The figure shows three views and two pictorial views of one solid part (mm, origin at its lowest corner). Answer the questions. A direction names the side the tool comes from. Coordinates: 2 decimals unless noted, no trailing zeros. Return JSON: item names as keys, results as strings. Group by question number.
1. A straight line is drawn through the part: L1, parallel to Y at x = 38, z = 5. Find the intervals that lie inside material, in ascending order. Write a range as from..to.
2. Which of the six approach directions +Z, -Z, +X, -X, +Y, -Y give full straight-line access (tool end or side, diameter ignored) to the marked faces 5 and 6?
3. Section A-A (z = 10.5) is taken. Count the separate pieces of the cut face and the enclosed holes in it, then the cut area to 3 significant figures.
4. Given P1, Ø1.6, axis at x = 18, y = 1, coming from the +Z side; P2, Ø5.5, axis at x = 38.1, y = 9.525, coming from the -Z side, each flat-ended and moving along its own axis, determine where each tip first touches the part or whether it passes through.
5. The mould has two halves that part along X. Classify the marked faces 1, 2, 3 and 4: pulls with the +X half, pulls with the -X half, needs draft (parallel to the pull), parting line crosses it, or undercut.
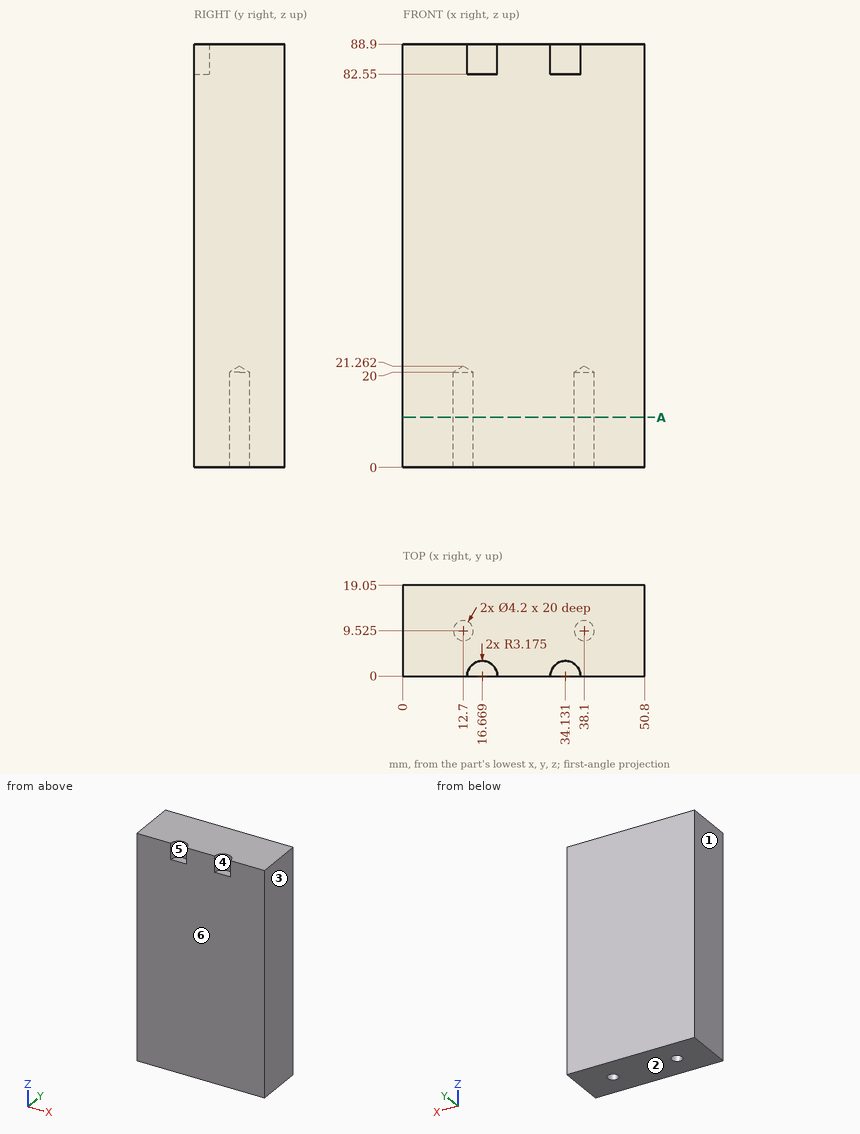
Worked out:
{
 "1": {"L1": "0..7.43, 11.62..19.05"},
 "2": {"face 5": "+Z, -Y", "face 6": "+Z, -Z, +X, -X, -Y"},
 "3": {"separate pieces": "1", "enclosed holes": "2", "area": "940 mm^2"},
 "4": {"P1": "z = 82.55", "P2": "z = 0"},
 "5": {"face 1": "pulls with the -X half", "face 2": "needs draft", "face 3": "pulls with the +X half", "face 4": "undercut"}
}
